Can you work these out from the model? Positions are in its coordinate system, mm. A direction names the side the tool comes from. Coordinates: 2 decimals unless noted, no trailing zeros. Order: outer loops, then holes, each group sorted by start corner. A loop starts at its lowest first (then second) coordinate and runs counter-clockwise, first axis right, second up. Notation, with made-up numbers: (32, -9.75) -> (60, -9.75) arc R28 ccw to (60, 20.25) -> close; hole circle Ø8 at (64, 6). An arc over 180 degrees is marked (long way). Use a Markdown table: item, result. Add a question column.
1. If I drill on line 1 along Y through (x, z) = (0, -2); line 2 along Y through (x, z) = (-15, -63); line 3 along X through (y, z) = (0, -39), over which ranges is the centre line in solid material (lowest first)? Write a range as from..to.
2. Suppose I cut it at C-C, the plane z = -57. List the corners of the cut face in (x, y) for me.
3. We'd pull the mould along X, two halves only. Please class faces 3 (the flat face through (-1, -11, -69)), 4 (the cylindrical face through (34.2, -5.9, -64.6)): pulls with the +X half, pulls with the -X half, needs draft (parallel to the pull), parting line crosses it, or undercut.
4. For pin 1 Ø7 at (x, z) = (8.5, -63) entering from +Y; pin 2 Ø2 at (x, z) = (-41.5, -23.5) entering from -Y; pin 3 Ø4 at (x, y) = (46.77, 27) entering from +Z; pin 4 Ø2.5 at (x, y) = (-15, -5) entering from -Z, each with a flat end and sliding along its axis, tell me the tip position at first contact or that it passes through.
5. Suppose I cut it at B-B, the plane y = 0. List the corners of the cut face in (x, z) for me.
6. For faces 1 (the flat face through (0, -54, -6)), 2 (the flat face through (9, -10, -65)), which set-ups out of +Z, -Z, +X, -X, +Y, -Y let a thin tool reach every point of the face, with its end or its side?
7. Suppose I cut it at D-D, the plane x = 33. State how many separate pieces and enclosed holes the cut face has, then the cut area to 3 significant figures.
8. Suppose I cut it at A-A, the plane x = 0. List the corners of the cut face in (y, z) for me, then the cut area to 3 significant figures.
```python
from build123d import *

# Parameters (mm, degrees)
SKETCH2_W          = 50
SKETCH2_H          = 9
SKETCH2_W_2        = 8
SKETCH2_H_2        = 60
SKETCH3_R          = 2.35
CUT_EXTRUDE1_DEPTH = 6
CUT_EXTRUDE2_REACH = 109.187
SKETCH4_R          = 1.5
SKETCH4_W          = 41
SKETCH4_H          = 20
FILLET1_R          = 10


with BuildPart() as part:
    # Sketch2 → Revolve1 (revolve)
    with BuildSketch(Plane(origin=(0, 0, 0), x_dir=(1, 0, 0), z_dir=(0, 1, 0))):
        with Locations((25, 64.5)):
            Rectangle(SKETCH2_W, SKETCH2_H)
        with Locations((54, 64.5)):
            Rectangle(SKETCH2_W_2, SKETCH2_H)
        with Locations((54, 30)):
            Rectangle(SKETCH2_W_2, SKETCH2_H_2)
    revolve(axis=Axis((0, 0, 1000), (0, 0, -1)))

    # Sketch3 → Cut-Extrude1 (cut)
    with BuildSketch(Plane.XY):
        with Locations((46.765371804, 27)):
            Circle(SKETCH3_R)
        with Locations((0, 54)):
            Circle(SKETCH3_R)
        with Locations((46.765371804, -27)):
            Circle(SKETCH3_R)
        with Locations((0, -54)):
            Circle(SKETCH3_R)
        with Locations((-46.765371804, -27)):
            Circle(SKETCH3_R)
        with Locations((-46.765371804, 27)):
            Circle(SKETCH3_R)
    extrude(amount=-CUT_EXTRUDE1_DEPTH, mode=Mode.SUBTRACT)

    # Sketch4 → Cut-Extrude2 (cut, up to next)
    with BuildSketch(Plane(origin=(0, 0, -69), x_dir=(-1, 0, 0), z_dir=(0, 0, -1)), mode=Mode.PRIVATE) as cut_extrude2_sk1:
        with Locations((15, 5)):
            Circle(SKETCH4_R)
    cut_extrude2_tool1 = extrude(cut_extrude2_sk1.sketch, amount=-CUT_EXTRUDE2_REACH, mode=Mode.PRIVATE) & part.part
    # Sketch4 → Cut-Extrude2 (cut, up to next)
    with BuildSketch(Plane(origin=(0, 0, -69), x_dir=(-1, 0, 0), z_dir=(0, 0, -1)), mode=Mode.PRIVATE) as cut_extrude2_sk2:
        with Locations((15, -5)):
            Circle(SKETCH4_R)
    cut_extrude2_tool2 = extrude(cut_extrude2_sk2.sketch, amount=-CUT_EXTRUDE2_REACH, mode=Mode.PRIVATE) & part.part
    # Sketch4 → Cut-Extrude2 (cut, up to next)
    with BuildSketch(Plane(origin=(0, 0, -69), x_dir=(-1, 0, 0), z_dir=(0, 0, -1)), mode=Mode.PRIVATE) as cut_extrude2_sk3:
        with Locations((-33, -5)):
            Circle(SKETCH4_R)
    cut_extrude2_tool3 = extrude(cut_extrude2_sk3.sketch, amount=-CUT_EXTRUDE2_REACH, mode=Mode.PRIVATE) & part.part
    # Sketch4 → Cut-Extrude2 (cut, up to next)
    with BuildSketch(Plane(origin=(0, 0, -69), x_dir=(-1, 0, 0), z_dir=(0, 0, -1)), mode=Mode.PRIVATE) as cut_extrude2_sk4:
        with Locations((-33, 5)):
            Circle(SKETCH4_R)
    cut_extrude2_tool4 = extrude(cut_extrude2_sk4.sketch, amount=-CUT_EXTRUDE2_REACH, mode=Mode.PRIVATE) & part.part
    # Sketch4 → Cut-Extrude2 (cut, up to next)
    with BuildSketch(Plane(origin=(0, 0, -69), x_dir=(-1, 0, 0), z_dir=(0, 0, -1)), mode=Mode.PRIVATE) as cut_extrude2_sk5:
        with Locations((-9, 0)):
            Rectangle(SKETCH4_W, SKETCH4_H)
    cut_extrude2_tool5 = extrude(cut_extrude2_sk5.sketch, amount=-CUT_EXTRUDE2_REACH, mode=Mode.PRIVATE) & part.part
    add(cut_extrude2_tool1.solids().sort_by_distance((-15, 5, -69))[0], mode=Mode.SUBTRACT)
    add(cut_extrude2_tool2.solids().sort_by_distance((-15, -5, -69))[0], mode=Mode.SUBTRACT)
    add(cut_extrude2_tool3.solids().sort_by_distance((33, -5, -69))[0], mode=Mode.SUBTRACT)
    add(cut_extrude2_tool4.solids().sort_by_distance((33, 5, -69))[0], mode=Mode.SUBTRACT)
    add(cut_extrude2_tool5.solids().sort_by_distance((9, 0, -69))[0], mode=Mode.SUBTRACT)

    # Fillet1
    fillet1_edges = [part.edges().sort_by_distance(p)[0] for p in [
        (-58, 0, -69),
    ]]
    fillet(fillet1_edges, radius=FILLET1_R)


solid = part.part
```
Worked out:
| question | item | result |
|---|---|---|
| 1 | line 1 | y = -58..-56.35, -51.65..-50, 50..51.65, 56.35..58 |
| 1 | line 2 | y = -55.16..-6.5, -3.5..3.5, 6.5..55.16 |
| 1 | line 3 | x = -58..-50, 50..58 |
| 2 | outline | circle Ø116 at (0, 0); hole circle Ø100 at (0, 0) |
| 3 | face 3 | needs draft |
| 3 | face 4 | undercut |
| 4 | pin 1 | stops at y = 57.57 |
| 4 | pin 2 | stops at y = -41.52 |
| 4 | pin 3 | stops at z = -6 |
| 4 | pin 4 | passes through |
| 5 | outline | (-58, -59) arc R10 ccw to (-48, -69) -> (-11.5, -69) -> (-11.5, -60) -> (-50, -60) -> (-50, 0) -> (-58, 0) -> close; (29.5, -69) -> (48, -69) arc R10 ccw to (58, -59) -> (58, 0) -> (50, 0) -> (50, -60) -> (29.5, -60) -> close |
| 6 | face 1 | +Z |
| 6 | face 2 | +Z, -Z |
| 7 | separate pieces | 3 |
| 7 | enclosed holes | 0 |
| 7 | area | 1,970 mm² |
| 8 | outline | (-58, -59) arc R10 ccw to (-48, -69) -> (-10, -69) -> (-10, -60) -> (-50, -60) -> (-50, 0) -> (-51.65, 0) -> (-51.65, -6) -> (-56.35, -6) -> (-56.35, 0) -> (-58, 0) -> close; (10, -69) -> (48, -69) arc R10 ccw to (58, -59) -> (58, 0) -> (56.35, 0) -> (56.35, -6) -> (51.65, -6) -> (51.65, 0) -> (50, 0) -> (50, -60) -> (10, -60) -> close |
| 8 | area | 1,720 mm² |
